For this review, use the dimensioned drawing (mm, ordinates from the lowest corner) and the shaded views. A direction names the side the tool comes from. Give positions to 0.01 mm unless a question says otherwise; leave off trailing zeros. Order: outer loops, then holes, each group sorted by start corner. A loop starts at its lowest first (then second) coordinate and runs counter-clockwise, first axis right, second up. Notation, with made-up numbers: (53.5, -12.75) -> (84.5, -12.75) arc R31 cw to (84.5, 14.25) -> close; hole circle Ø1 at (48, 75.5). An arc over 180 degrees is marked (long way). One line per item, written item: value. Start each with the question number.
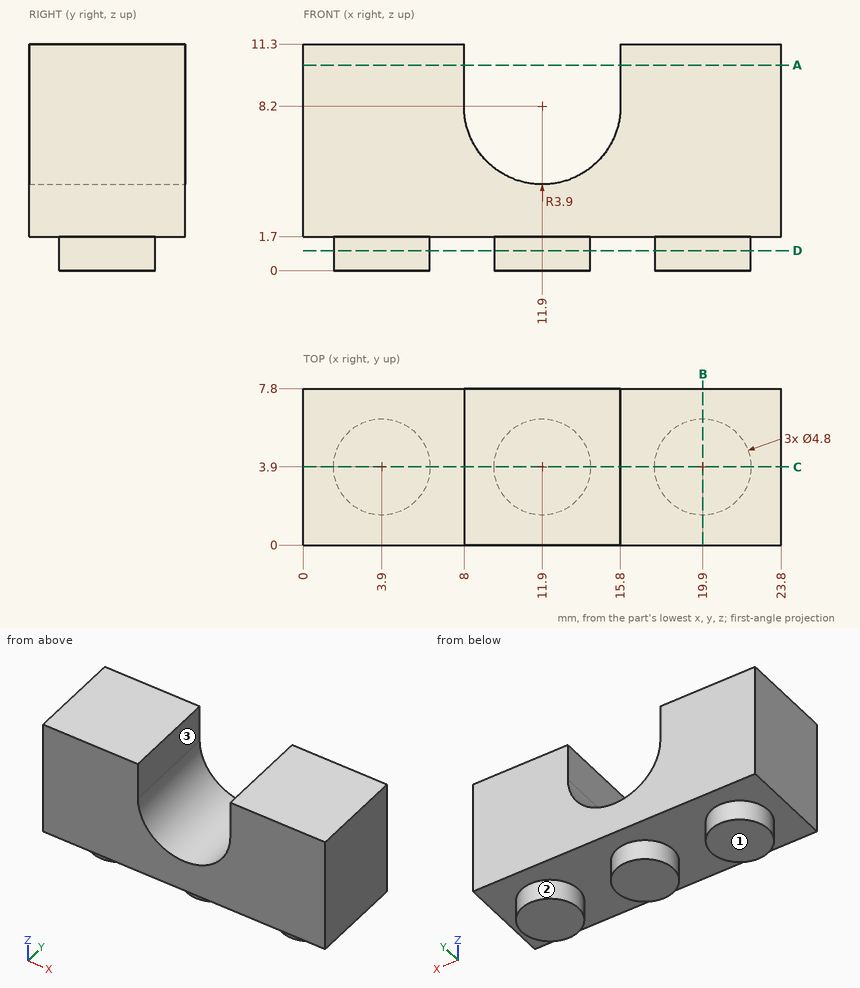
Q1. For the marked faces 1, 2 and 3, list the 3-axis set-ups (+Z, -Z, +X, -X, +Y, -Y) from which the entire face can be reached by the end or side of a thin tool; tool diameter is ignored.
Q2. Take a section at B-B (x = 19.9). State the section outline as (y, z) points, and give its area (3 significant figures).
Q3. For line 1 along X through (y, z) = (2.75, 10); line 2 along Z through (x, y) = (6.25, 2.5); line 3 along X through (y, z) = (0.75, 5.5), list the stretches that pass through material, from the lowest coordinate up.
Q4. Take a section at D-D (z = 1). State the section outline as (x, y) points, and give its area (3 significant figures).
Q5. Take a section at A-A (z = 10.25). State the section outline as (x, y) points.
Q6. Take a section at C-C (y = 3.9). State the section outline as (x, z) points, and give its area (3 significant figures).
Q7. For pin 1 Ø2 at (x, y) = (17, 6) entering from -Z, flat-tipped, find the tip position at first contact; note if it passes through.
Answers below:
1. face 1: -Z, +X, -X, +Y, -Y
1. face 2: -Z
1. face 3: +Z, +Y, -Y
2. outline: (0, 1.7) -> (1.5, 1.7) -> (1.5, 0) -> (6.3, 0) -> (6.3, 1.7) -> (7.8, 1.7) -> (7.8, 11.3) -> (0, 11.3) -> close
2. area: 83.0 mm²
3. line 1: x = 0 to 8, 15.8 to 23.8
3. line 2: z = 1.7 to 11.3
3. line 3: x = 0 to 9.09, 14.71 to 23.8
4. outline: circle Ø4.8 at (3.9, 3.9); circle Ø4.8 at (11.9, 3.9); circle Ø4.8 at (19.9, 3.9)
4. area: 54.3 mm²
5. outline: (0, 0) -> (8, 0) -> (8, 7.8) -> (0, 7.8) -> close; (15.8, 0) -> (23.8, 0) -> (23.8, 7.8) -> (15.8, 7.8) -> close
6. outline: (0, 1.7) -> (1.5, 1.7) -> (1.5, 0) -> (6.3, 0) -> (6.3, 1.7) -> (9.5, 1.7) -> (9.5, 0) -> (14.3, 0) -> (14.3, 1.7) -> (17.5, 1.7) -> (17.5, 0) -> (22.3, 0) -> (22.3, 1.7) -> (23.8, 1.7) -> (23.8, 11.3) -> (15.8, 11.3) -> (15.8, 8.2) arc R3.9 cw to (8, 8.2) -> (8, 11.3) -> (0, 11.3) -> close
6. area: 205 mm²
7. pin 1: stops at z = 1.7
